from build123d import *

# Parameters (mm, degrees)
SKETCH1_R                      = 44.45
SKETCH1_R_2                    = 3.25
BOSS_EXTRUDE1_DEPTH            = 3.175
BOSS_EXTRUDE2_DEPTH            = 25.4
CBORE_FOR_M6_SHCS2_D           = 7
CBORE_FOR_M6_SHCS2_CBORE_D     = 11
CBORE_FOR_M6_SHCS2_CBORE_DEPTH = 6
SKETCH10_W                     = 206.275362682
SKETCH10_H                     = 234.398565581
CUT_EXTRUDE1_DEPTH             = 15.2875
CUT_EXTRUDE1_DEPTH_BACK        = 10.16


with BuildPart() as part:
    # Sketch1 → Boss-Extrude1 (new body)
    with BuildSketch(Plane(origin=(0, 0, 0), x_dir=(1, 0, 0), z_dir=(0, 1, 0))):
        with BuildLine():
            Line((-57.15, 63.5), (57.15, 63.5))
            ThreePointArc((57.15, 63.5), (61.640128061, 61.640128061), (63.5, 57.15))
            Line((63.5, 57.15), (63.5, -57.15))
            ThreePointArc((63.5, -57.15), (61.640128061, -61.640128061), (57.15, -63.5))
            Line((57.15, -63.5), (-57.15, -63.5))
            ThreePointArc((-57.15, -63.5), (-61.640128061, -61.640128061), (-63.5, -57.15))
            Line((-63.5, -57.15), (-63.5, 57.15))
            ThreePointArc((-63.5, 57.15), (-61.640128061, 61.640128061), (-57.15, 63.5))
        make_face()
        Circle(SKETCH1_R, mode=Mode.SUBTRACT)
        with Locations((-57.15, 53.975)):
            Circle(SKETCH1_R_2, mode=Mode.SUBTRACT)
        with Locations((57.15, 53.975)):
            Circle(SKETCH1_R_2, mode=Mode.SUBTRACT)
        with Locations((57.15, -53.975)):
            Circle(SKETCH1_R_2, mode=Mode.SUBTRACT)
        with Locations((-57.15, -53.975)):
            Circle(SKETCH1_R_2, mode=Mode.SUBTRACT)
    extrude(amount=BOSS_EXTRUDE1_DEPTH)

    # Sketch3 → Boss-Extrude2 (add)
    with BuildSketch(Plane(origin=(0, 3.175, 0), x_dir=(1, 0, 0), z_dir=(0, 1, 0))):
        with BuildLine():
            Line((-57.15, -63.5), (57.15, -63.5))
            ThreePointArc((57.15, -63.5), (61.640128061, -61.640128061), (63.5, -57.15))
            Line((63.5, -57.15), (63.5, 57.15))
            ThreePointArc((63.5, 57.15), (61.640128061, 61.640128061), (57.15, 63.5))
            Line((57.15, 63.5), (-57.15, 63.5))
            ThreePointArc((-57.15, 63.5), (-61.640128061, 61.640128061), (-63.5, 57.15))
            Line((-63.5, 57.15), (-63.5, -57.15))
            ThreePointArc((-63.5, -57.15), (-61.640128061, -61.640128061), (-57.15, -63.5))
        make_face()
        with BuildLine():
            Line((-54.700256121, 45.358975516), (-45.358975516, 54.700256121))
            ThreePointArc((-45.358975516, 54.700256121), (-41.238798986, 57.453270063), (-36.378719395, 58.42))
            Line((-36.378719395, 58.42), (36.378719395, 58.42))
            ThreePointArc((36.378719395, 58.42), (41.238798986, 57.453270063), (45.358975516, 54.700256121))
            Line((45.358975516, 54.700256121), (54.700256121, 45.358975516))
            ThreePointArc((54.700256121, 45.358975516), (57.453270063, 41.238798986), (58.42, 36.378719395))
            Line((58.42, 36.378719395), (58.42, -36.378719395))
            ThreePointArc((58.42, -36.378719395), (57.453270063, -41.238798986), (54.700256121, -45.358975516))
            Line((54.700256121, -45.358975516), (45.358975516, -54.700256121))
            ThreePointArc((45.358975516, -54.700256121), (41.238798986, -57.453270063), (36.378719395, -58.42))
            Line((36.378719395, -58.42), (-36.378719395, -58.42))
            ThreePointArc((-36.378719395, -58.42), (-41.238798986, -57.453270063), (-45.358975516, -54.700256121))
            Line((-45.358975516, -54.700256121), (-54.700256121, -45.358975516))
            ThreePointArc((-54.700256121, -45.358975516), (-57.453270063, -41.238798986), (-58.42, -36.378719395))
            Line((-58.42, -36.378719395), (-58.42, 36.378719395))
            ThreePointArc((-58.42, 36.378719395), (-57.453270063, 41.238798986), (-54.700256121, 45.358975516))
        make_face(mode=Mode.SUBTRACT)
    extrude(amount=BOSS_EXTRUDE2_DEPTH)

    # CBORE for M6 SHCS2 (through all)
    with Locations(Plane(origin=(0, 0, 0), x_dir=(-1, 0, 0), z_dir=(0, -1, 0))):
        with Locations((-55.88, 55.88), (55.88, 55.88), (55.88, -55.88), (-55.88, -55.88)):
            CounterBoreHole(CBORE_FOR_M6_SHCS2_D / 2, CBORE_FOR_M6_SHCS2_CBORE_D / 2, CBORE_FOR_M6_SHCS2_CBORE_DEPTH)

    # Sketch10 → Cut-Extrude1 (cut, two sides)
    with BuildSketch(Plane(origin=(0, 14.2875, 0), x_dir=(-1, 0, 0), z_dir=(0, -1, 0))) as cut_extrude1_sk:
        with Locations((4.587579463, 2.84706708)):
            Rectangle(SKETCH10_W, SKETCH10_H)
    extrude(amount=CUT_EXTRUDE1_DEPTH, mode=Mode.SUBTRACT)
    extrude(cut_extrude1_sk.sketch, amount=-CUT_EXTRUDE1_DEPTH_BACK, mode=Mode.SUBTRACT)


solid = part.part
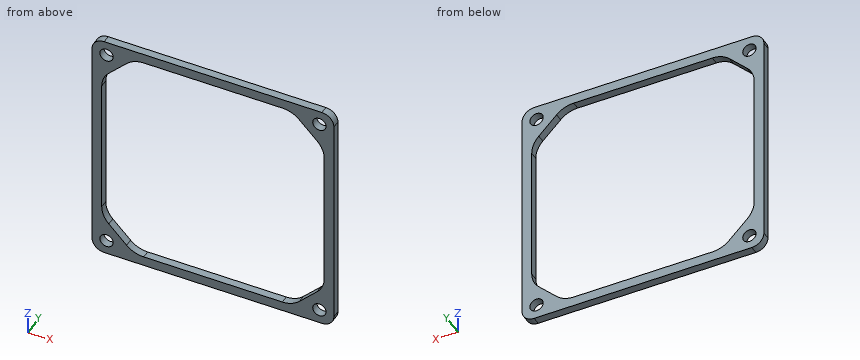
Could you check a few things on this model? Use its own coordinates, in mm. Give positions to 0.01 mm unless a question says otherwise; leave off trailing zeros. Order: outer loops, then holes, each group sorted by start corner. A loop starts at its lowest first (then second) coordinate and runs counter-clockwise, first axis right, second up. Notation, with made-up numbers: (10, 52) - (43, 52) arc R20 cw to (43, 62) - close; hole circle Ø11 at (-15, -31). An arc over 180 degrees is marked (long way). One line per item, written item: value. Start each with the question number.
1. If I drill on probe 1 along X at (y, z) = (25.2, -14.5); probe 2 along X at (y, z) = (26.85, -55.88); probe 3 along Z at (x, y) = (-57, 27.4), over which ranges is the centre line in solid material (lowest first)?
2. Imagine slicing it at A-A on x = -30.5. List the corners of the cut face in (y, z) for me (1 decimal), plus the area to 3 significant figures.
3. For P1, Ø6.5, axis at x = 55.88, z = -55.88, coming from the -Y side; P2, Ø9, axis at x = 55.88, z = 55.88, coming from the +Y side (3 decimals), each with a flat end and sliding along its axis, tell me the tip position at first contact or that it passes through.
4. Imagine slicing it at B-B on y = 27.9. List the corners of the cut face in (x, z) for me.
5. Imagine slicing it at C-C on z = -10.5. List the corners of the cut face in (x, y) for me (1 decimal).
Values:
1. probe 1: -63.5 to -58.42, 58.42 to 63.5
1. probe 2: -63.5 to -59.38, -52.38 to -44, 44 to 52.38, 59.38 to 63.5
1. probe 3: -63.5 to -59.2, -52.56 to -42.21, 42.21 to 52.56, 59.2 to 63.5
2. outline: (24.4, -63.5) - (28.6, -63.5) - (28.6, -58.4) - (24.4, -58.4) - close; (24.4, 58.4) - (28.6, 58.4) - (28.6, 63.5) - (24.4, 63.5) - close
2. area: 41.9 mm²
3. P1: through
3. P2: y = 28.575
4. outline: (-63.5, -57.15) arc R6.35 ccw to (-57.15, -63.5) - (57.15, -63.5) arc R6.35 ccw to (63.5, -57.15) - (63.5, 57.15) arc R6.35 ccw to (57.15, 63.5) - (-57.15, 63.5) arc R6.35 ccw to (-63.5, 57.15) - close; hole circle Ø7 at (-55.88, -55.88); hole circle Ø7 at (-55.88, 55.88); hole (-58.42, -36.38) arc R12.7 ccw to (-54.7, -45.36) - (-45.36, -54.7) arc R12.7 ccw to (-36.38, -58.42) - (36.38, -58.42) arc R12.7 ccw to (45.36, -54.7) - (54.7, -45.36) arc R12.7 ccw to (58.42, -36.38) - (58.42, 36.38) arc R12.7 ccw to (54.7, 45.36) - (45.36, 54.7) arc R12.7 ccw to (36.38, 58.42) - (-36.38, 58.42) arc R12.7 ccw to (-45.36, 54.7) - (-54.7, 45.36) arc R12.7 ccw to (-58.42, 36.38) - close; hole circle Ø7 at (55.88, -55.88); hole circle Ø7 at (55.88, 55.88)
5. outline: (-63.5, 24.4) - (-58.4, 24.4) - (-58.4, 28.6) - (-63.5, 28.6) - close; (58.4, 24.4) - (63.5, 24.4) - (63.5, 28.6) - (58.4, 28.6) - close
